from build123d import *

# Parameters (mm, degrees)
PAD_DEPTH       = 34
SKETCH002_W     = 21.5
SKETCH002_H     = 30.5
POCKET_DEPTH    = 21.5
POCKET001_DEPTH = 5
POCKET002_DEPTH = 5
SKETCH004_W     = 2
SKETCH004_H     = 34
PAD001_DEPTH    = 8
SKETCH005_R     = 2
POCKET003_DEPTH = 5
CHAMFER_SIZE    = 1
SKETCH006_W     = 2
SKETCH006_H     = 34
PAD002_DEPTH    = 8
SKETCH007_R     = 2
POCKET004_DEPTH = 5
CHAMFER001_SIZE = 1
FILLET_R        = 1


with BuildPart() as part:
    # Sketch → Pad (new body)
    with BuildSketch(Plane.YZ):
        with BuildLine():
            Line((-11.011805, 9.998219), (10.488195, 9.998219))
            ThreePointArc((12.238195, 8.248219), (11.725632, 9.485655), (10.488195, 9.998219))
            Line((12.238195, 8.248219), (12.238195, -12.001781))
            Line((12.238195, -12.001781), (-12.761805, -12.001781))
            Line((-12.761805, -12.001781), (-12.761805, 8.248219))
            ThreePointArc((-11.011805, 9.998219), (-12.249242, 9.485655), (-12.761805, 8.248219))
        make_face()
    extrude(amount=PAD_DEPTH)

    # Sketch002 (on Face2 of Pad) → Pocket (cut)
    with BuildSketch(Plane.YX.offset(12.001781)):
        with Locations((-0.261805, 17)):
            Rectangle(SKETCH002_W, SKETCH002_H)
    extrude(amount=-POCKET_DEPTH, mode=Mode.SUBTRACT)

    # Sketch001 (on Face7 of Pad) → Pocket001 (cut)
    with BuildSketch(Plane(origin=(0, 0, 0), x_dir=(0, 1, 0), z_dir=(-1, 0, 0))):
        with BuildLine():
            Line((7.488195, 12.001781), (-8.011805, 12.001781))
            Line((-8.011805, 12.001781), (-8.011805, -2.498219))
            ThreePointArc((-8.011805, -2.498219), (-7.718912, -3.205325), (-7.011805, -3.498219))
            Line((-7.011805, -3.498219), (6.488195, -3.498219))
            ThreePointArc((6.488195, -3.498219), (7.195302, -3.205325), (7.488195, -2.498219))
            Line((7.488195, -2.498219), (7.488195, 12.001781))
        make_face()
    extrude(amount=-POCKET001_DEPTH, mode=Mode.SUBTRACT)

    # Sketch003 (on Face5 of Pocket001) → Pocket002 (cut)
    with BuildSketch(Plane.YZ.offset(34)):
        with BuildLine():
            Line((-6.261805, -12.001781), (5.738195, -12.001781))
            Line((5.738195, -12.001781), (5.738195, 2.998219))
            ThreePointArc((5.738195, 2.998219), (5.445302, 3.705325), (4.738195, 3.998219))
            Line((4.738195, 3.998219), (-5.261805, 3.998219))
            ThreePointArc((-5.261805, 3.998219), (-5.968912, 3.705325), (-6.261805, 2.998219))
            Line((-6.261805, 2.998219), (-6.261805, -12.001781))
        make_face()
    extrude(amount=-POCKET002_DEPTH, mode=Mode.SUBTRACT)

    # Sketch004 (on Face17 of Pocket002) → Pad001 (join)
    with BuildSketch(Plane(origin=(0, -12.761805, 0), x_dir=(0, 0, -1), z_dir=(0, -1, 0))):
        with Locations((11.001781, 17)):
            Rectangle(SKETCH004_W, SKETCH004_H)
    extrude(amount=PAD001_DEPTH)

    # Sketch005 (on Face28 of Pad001) → Pocket003 (cut)
    with BuildSketch(Plane(origin=(0, 0, -10.001781), x_dir=(0, -1, 0), z_dir=(0, 0, 1))):
        with Locations((16.761805, 30)):
            Circle(SKETCH005_R)
        with Locations((16.761805, 4)):
            Circle(SKETCH005_R)
    extrude(amount=-POCKET003_DEPTH, mode=Mode.SUBTRACT)

    # Chamfer
    chamfer_edges = [part.edges().sort_by_distance(p)[0] for p in [
        (4, -14.761805, -10.001781),
        (30, -14.761805, -10.001781),
    ]]
    chamfer(chamfer_edges, length=CHAMFER_SIZE)

    # Sketch006 (on Face15 of Chamfer) → Pad002 (join)
    with BuildSketch(Plane.ZX.offset(12.238195)):
        with Locations((-11.001781, 17)):
            Rectangle(SKETCH006_W, SKETCH006_H)
    extrude(amount=PAD002_DEPTH)

    # Sketch007 (on Face34 of Pad002) → Pocket004 (cut)
    with BuildSketch(Plane(origin=(0, 0, -10.001781), x_dir=(0, -1, 0), z_dir=(0, 0, 1))):
        with Locations((-16.238195, 30)):
            Circle(SKETCH007_R)
        with Locations((-16.238195, 4)):
            Circle(SKETCH007_R)
    extrude(amount=-POCKET004_DEPTH, mode=Mode.SUBTRACT)

    # Chamfer001
    chamfer001_edges = [part.edges().sort_by_distance(p)[0] for p in [
        (30, 18.238195, -10.001781),
        (4, 18.238195, -10.001781),
    ]]
    chamfer(chamfer001_edges, length=CHAMFER001_SIZE)

    # Fillet
    fillet_edges = [part.edges().sort_by_distance(p)[0] for p in [
        (0, -20.761805, -11.001781),
        (34, -20.761805, -11.001781),
        (0, 20.238195, -11.001781),
        (34, 20.238195, -11.001781),
    ]]
    fillet(fillet_edges, radius=FILLET_R)


solid = part.part
Geometry: final body of the model. Coordinates: model frame, mm. A direction names the side the tool comes from. Coordinates: 2 decimals unless noted, no trailing zeros. Order: outer loops, then holes, each group sorted by start corner. A loop starts at its lowest first (then second) coordinate and runs counter-clockwise, first axis right, second up.
1) First-contact query: P1, Ø6.5, axis at x = 16.5, z = -5, coming from the +Y side; P2, Ø4, axis at x = 19.5, y = 15, coming from the +Z side; P3, Ø1.4, axis at x = 0.5, z = -6, coming from the -Y side; P4, Ø3.5, axis at x = 4, y = 16.24, coming from the +Z side. Flat tips, straight axial feed; report the tip coordinate or a pass-through.
Result sheet:
P1: stops at y = 12.24
P2: stops at z = -10
P3: stops at y = -12.76
P4: passes through
2) Set-up query: faces 1 (the flat face through (17, 12.238, -1)), 2 (the cylindrical face through (0.3, 19.95, -10.99)), 3 (the cylindrical face through (33.14, 5.45, 3.7)), 4 (the flat face through (17, -12.762, -1)). Return all of +Z, -Z, +X, -X, +Y, -Y with unobstructed straight access to the full face (end or side cutting, diameter ignored); none if empty.
Result sheet:
face 1: +Z, +X, -X, +Y
face 2: +Z, -Z, -X, +Y
face 3: -Z, +X
face 4: +Z, +X, -X, -Y
3) Ray query, probe 1 along Y at (x, z) = (19, -8.75); probe 2 along X at (y, z) = (-1, 5); probe 3 along Z at (x, y) = (33.5, 17.5). Return the intervals inside material, ascending.
Result sheet:
probe 1: y = -12.76 to -11.01, 10.49 to 12.24
probe 2: x = 0 to 1.75, 32.25 to 34
probe 3: z = -12 to -10
4) Section C-C (z = 0.25). Return loops of the section in (x, y), then the cut area to 3 significant figures.
Result sheet:
outline: (0, -12.76) - (34, -12.76) - (34, -6.26) - (32.25, -6.26) - (32.25, -11.01) - (1.75, -11.01) - (1.75, -8.01) - (0, -8.01) - close; (0, 7.49) - (1.75, 7.49) - (1.75, 10.49) - (32.25, 10.49) - (32.25, 5.74) - (34, 5.74) - (34, 12.24) - (0, 12.24) - close
area: 146 mm2
5) Section B-B (z = 4.75). Return loops of the section in (x, y), then the cut area to 3 significant figures.
Result sheet:
outline: (0, -12.76) - (34, -12.76) - (34, 12.24) - (0, 12.24) - close; hole (1.75, -11.01) - (32.25, -11.01) - (32.25, 10.49) - (1.75, 10.49) - close
area: 194 mm2
6) Section A-A (x = 30). Return loops of the section in (y, z), then the cut area to 3 significant figures.
Result sheet:
outline: (-20.76, -12) - (-18.76, -12) - (-18.76, -11) - (-19.76, -10) - (-20.76, -10) - close; (-14.76, -12) - (-11.01, -12) - (-11.01, 9.5) - (10.49, 9.5) - (10.49, -12) - (14.24, -12) - (14.24, -11) - (13.24, -10) - (12.24, -10) - (12.24, 8.25) arc R1.75 ccw to (10.49, 10) - (-11.01, 10) arc R1.75 ccw to (-12.76, 8.25) - (-12.76, -10) - (-13.76, -10) - (-14.76, -11) - close; (18.24, -12) - (20.24, -12) - (20.24, -10) - (19.24, -10) - (18.24, -11) - close
area: 100 mm2
7) Section D-D (y = -3). Return loops of the section in (x, z), then the cut area to 3 significant figures.
Result sheet:
outline: (0, 3.5) - (1.75, 3.5) - (1.75, 9.5) - (32.25, 9.5) - (32.25, 4) - (34, 4) - (34, 10) - (0, 10) - close
area: 37.1 mm2
8) Draft query along Y for faces 5 (the flat face through (33, -6.262, -4)), 6 (the cylindrical face through (33.7, 19.95, -10.99)), 7 (the flat face through (1, 7.488, -5)), 8 (the flat face through (17, -20.762, -11)). Return one class per face: released by +Y, released by -Y, zero draft, split by the parting line, or undercut.
Result sheet:
face 5: undercut
face 6: released by +Y
face 7: undercut
face 8: released by -Y
